Work out the finished part from the listing and answer in its coordinate system (mm). A direction names the side the tool comes from. Round coordinates to 2 decimals unless told otherwise and drop trailing zeros. Order: outer loops, then holes, each group sorted by start corner. A loop starts at its lowest first (then second) coordinate and runs counter-clockwise, first axis right, second up. Notation, with made-up numbers: M -5.5,28 L 7.5,28 A4 ccw 7.5,34 Z; hole C -39,-22.75 d8. An arc over 180 degrees is marked long. Answer as a JSON object with one key per item and string values. Group by question number.
from build123d import *

# Parameters (mm, degrees)
F1_DEPTH = 3
F0_R     = 3
F2_DEPTH = 11.6


with BuildPart() as f1:
    # F0 (on Top) → F1 (new body)
    with BuildSketch(Plane.XY):
        with BuildLine():
            Line((-15.406721, -12.5), (-15.406721, -7.5))
            Line((-15.406721, -7.5), (-28.609985, -11.163855))
            ThreePointArc((-28.609985, -11.163855), (-24.683184, -11.917774), (-22.906721, -15.5))
            ThreePointArc((-22.906721, -15.5), (-23.608966, -17.91393), (-25.496524, -19.57445))
            Line((-25.496524, -19.57445), (-10.406721, -12.5))
            Line((-10.406721, -12.5), (-15.406721, -12.5))
        make_face()
        Polygon((14.593279, 12.5), (-10.406721, 12.5), (-15.406721, 12.5), (-15.406721, 7.5), (-15.406721, -7.5), (-15.406721, -12.5), (-10.406721, -12.5), (14.593279, -12.5), (19.593279, -12.5), (19.593279, -7.5), (19.593279, 7.5), (19.593279, 12.5), align=None)
        with BuildLine():
            ThreePointArc((-25.496524, 19.57445), (-23.608966, 17.91393), (-22.906721, 15.5))
            ThreePointArc((-22.906721, 15.5), (-24.683184, 11.917774), (-28.609985, 11.163855))
            Line((-28.609985, 11.163855), (-15.406721, 7.5))
            Line((-15.406721, 7.5), (-15.406721, 12.5))
            Line((-15.406721, 12.5), (-10.406721, 12.5))
            Line((-10.406721, 12.5), (-25.496524, 19.57445))
        make_face()
        with BuildLine():
            Line((27.330159, -13.427958), (19.593279, -7.5))
            Line((19.593279, -7.5), (19.593279, -12.5))
            Line((19.593279, -12.5), (14.593279, -12.5))
            Line((14.593279, -12.5), (21.225295, -19.984407))
            ThreePointArc((21.225295, -19.984407), (21.299902, -13.93346), (27.330159, -13.427958))
        make_face()
        with BuildLine():
            Line((21.225295, 19.984407), (14.593279, 12.5))
            Line((14.593279, 12.5), (19.593279, 12.5))
            Line((19.593279, 12.5), (19.593279, 7.5))
            Line((19.593279, 7.5), (27.330159, 13.427958))
            ThreePointArc((27.330159, 13.427958), (21.299902, 13.93346), (21.225295, 19.984407))
        make_face()
    extrude(amount=F1_DEPTH)

    # F0 (on Top) → F2 (join)
    with BuildSketch(Plane.XY):
        with BuildLine():
            ThreePointArc((-22.906721, -15.5), (-24.683184, -11.917774), (-28.609985, -11.163855))
            ThreePointArc((-28.609985, -11.163855), (-31.626848, -17.06222), (-25.496524, -19.57445))
            ThreePointArc((-25.496524, -19.57445), (-23.608966, -17.91393), (-22.906721, -15.5))
        make_face()
        with Locations((-27.406721, -15.5)):
            Circle(F0_R, mode=Mode.SUBTRACT)
        with BuildLine():
            ThreePointArc((29.093279, -17), (28.628496, -15.008262), (27.330159, -13.427958))
            ThreePointArc((27.330159, -13.427958), (21.299902, -13.93346), (21.225295, -19.984407))
            ThreePointArc((21.225295, -19.984407), (26.189223, -21.207489), (29.093279, -17))
        make_face()
        with Locations((24.593279, -17)):
            Circle(F0_R, mode=Mode.SUBTRACT)
        with BuildLine():
            ThreePointArc((29.093279, 17), (26.189223, 21.207489), (21.225295, 19.984407))
            ThreePointArc((21.225295, 19.984407), (21.299902, 13.93346), (27.330159, 13.427958))
            ThreePointArc((27.330159, 13.427958), (28.628496, 15.008262), (29.093279, 17))
        make_face()
        with Locations((24.593279, 17)):
            Circle(F0_R, mode=Mode.SUBTRACT)
        with BuildLine():
            ThreePointArc((-28.609985, 11.163855), (-24.683184, 11.917774), (-22.906721, 15.5))
            ThreePointArc((-22.906721, 15.5), (-23.608966, 17.91393), (-25.496524, 19.57445))
            ThreePointArc((-25.496524, 19.57445), (-31.626848, 17.06222), (-28.609985, 11.163855))
        make_face()
        with Locations((-27.406721, 15.5)):
            Circle(F0_R, mode=Mode.SUBTRACT)
    extrude(amount=F2_DEPTH)


solid = f1.part
Item 1: Find section B-B (x = 23). Give the vertices of the cut face in (y, z).
Item 2: Each of these flat-tipped pins is pushed along its axis until it touches: pin 1 (3.5 mm diameter, centred on x = 7.5, z = 2, fed in from -Y); pin 2 (4 mm diameter, centred on y = -7.5, z = 7, fed in from +X); pin 3 (1.5 mm diameter, centred on x = -12.5, y = -8, fed in from +Z); pin 4 (1.5 mm diameter, centred on x = 2, z = 2, fed in from +Y). Where does it stop, or does it pass through?
Item 3: Find section D-D (y = -1). Give the vertices of the cut face in (x, z), and give its area (3 significant figures).
Item 4: A tool of negligible diameter and unlimited length cuts with its end or side. For faces 5 (the flat face through (-24, -16, 11.6)), 6 (the cylindrical face through (-29.787, 13.675, 5.719)), 7 (the flat face through (-18.06, -16.09, 1.48)), 8 (the flat face through (17.956, 16.295, 1.479)), 9 (the flat face through (19.593, 0, 1)), from which of +Z, -Z, +X, -X, +Y, -Y can it reach the whole face along a straight path? Write none if from no direction.
Item 5: Find section A-A (z = 7.75). Give the vertices of the cut face in (x, y).
Item 6: Consider L1, parallel to Y at x = 24, z = 3.75; L2, parallel to Y at x = -26, z = 6.5; L3, parallel to Y at x = -1.5, z = 2. Determine where each line is inside the solid, lowest interval first.
Item 7: Find section C-C (x = 5). Give the vertices of the cut face in (y, z).
Item 8: The mould has two halves that part along X. Classify faces 1 (the flat face through (-17.85, 15.99, 1.48)), 2 (the flat face through (23.408, 10.422, 1.479)), 3 (the flat face through (-22.101, 9.358, 1.479)), 4 (the flat face through (2, -12.5, 1)): +X half, -X half, draft (parallel to the pull), parting line (faces both ways), or undercut.
Responses:
{
 "1": {"outline": "M -21.21,0 L -19.54,0 L -19.54,11.6 L -21.21,11.6 Z; M -14.46,0 L -10.11,0 L -10.11,3 L -12.79,3 L -12.79,11.6 L -14.46,11.6 Z; M 10.11,0 L 14.46,0 L 14.46,11.6 L 12.79,11.6 L 12.79,3 L 10.11,3 Z; M 19.54,0 L 21.21,0 L 21.21,11.6 L 19.54,11.6 Z"},
 "2": {"pin 1": "stops at y = -12.5", "pin 2": "passes through", "pin 3": "stops at z = 3", "pin 4": "stops at y = 12.5"},
 "3": {"outline": "M -15.41,0 L 19.59,0 L 19.59,3 L -15.41,3 Z", "area": "105 mm^2"},
 "4": {"face 5": "+Z, +X, -X, +Y, -Y", "face 6": "+Z, -Z", "face 7": "+Z, -Z, -Y", "face 8": "+Z, -Z, +Y", "face 9": "+Z, -Z, +X"},
 "5": {"outline": "M -25.5,-19.57 A4.5 ccw -22.91,-15.5 A4.5 ccw long Z; M -25.5,19.57 A4.5 ccw long -22.91,15.5 A4.5 ccw Z; M 27.33,-13.43 A4.5 ccw long 29.09,-17 A4.5 ccw Z; M 27.33,13.43 A4.5 ccw 29.09,17 A4.5 ccw long Z; hole C -27.41,-15.5 d6; hole C -27.41,15.5 d6; hole C 24.59,-17 d6; hole C 24.59,17 d6"},
 "6": {"L1": "y = -21.46 to -19.94, -14.06 to -12.54, 12.54 to 14.06, 19.94 to 21.46", "L2": "y = -19.77 to -18.15, -12.85 to -11.23, 11.23 to 12.85, 18.15 to 19.77", "L3": "y = -12.5 to 12.5"},
 "7": {"outline": "M -12.5,0 L 12.5,0 L 12.5,3 L -12.5,3 Z"},
 "8": {"face 1": "undercut", "face 2": "+X half", "face 3": "-X half", "face 4": "undercut"}
}
